from build123d import *

# Parameters (mm, degrees)
F0_W     = 69.85
F0_H     = 101.6
F0_R     = 25.4
F1_DEPTH = 12.7
F2_W     = 69.85
F2_H     = 6.35
F3_DEPTH = 2.54


with BuildPart() as f1:
    # F0 (on Top) → F1 (new body)
    with BuildSketch(Plane.XY):
        Rectangle(F0_W, F0_H)
        Circle(F0_R, mode=Mode.SUBTRACT)
    extrude(amount=F1_DEPTH)

    # F2 (on face) → F3 (cut)
    with BuildSketch(Plane.XY.offset(12.7)):
        with BuildLine():
            Line((-24.8187093164, 5.4029314144), (-34.925, 5.4029314144))
            Line((-34.925, 5.4029314144), (-34.925, 0.3229314144))
            Line((-34.925, 0.3229314144), (-25.3989142655, 0.2348491713))
            ThreePointArc((-25.3989142655, 0.2348491713), (-25.2414282098, 2.8337787368), (-24.8187093164, 5.4029314144))
        make_face()
        with BuildLine():
            Line((-25.3989142655, 0.2348491713), (-34.925, 0.3229314144))
            Line((-34.925, 0.3229314144), (-34.925, -4.7570685856))
            Line((-34.925, -4.7570685856), (-24.9505570774, -4.7570685856))
            ThreePointArc((-24.9505570774, -4.7570685856), (-25.2981644957, -2.2721956671), (-25.3989142655, 0.2348491713))
        make_face()
        with BuildLine():
            Line((34.925, -0.3229314144), (34.925, 5.4029314144))
            Line((34.925, 5.4029314144), (24.8187093164, 5.4029314144))
            ThreePointArc((24.8187093164, 5.4029314144), (25.2542592114, 2.7170557009), (25.4, 0))
            ThreePointArc((25.4, 0), (25.3997285649, -0.1174258405), (25.3989142655, -0.2348491713))
            Line((25.3989142655, -0.2348491713), (34.925, -0.3229314144))
        make_face()
        with BuildLine():
            Line((34.925, -4.7570685856), (34.925, -0.3229314144))
            Line((34.925, -0.3229314144), (25.3989142655, -0.2348491713))
            ThreePointArc((25.3989142655, -0.2348491713), (25.2760743241, -2.5060061383), (24.9505570774, -4.7570685856))
            Line((24.9505570774, -4.7570685856), (34.925, -4.7570685856))
        make_face()
        with Locations((0, 36.0342099249)):
            Rectangle(F2_W, F2_H)
    extrude(amount=-F3_DEPTH, mode=Mode.SUBTRACT)


solid = f1.part
Verification items for the finished model (mm, model axes). A direction names the side the tool comes from. Give positions to 0.01 mm unless a question says otherwise; leave off trailing zeros. Write each loop counter-clockwise with the first axis right and the second up, starting at its lowest first coordinate (ties: lowest second). Pieces come first, ordered by that corner, then holes. Notation, with made-up numbers: M 22.25,29 L 46.25,29 A16 ccw 46.25,38 Z; hole C 19,32 d3. An arc over 180 degrees is marked long. Put each result on its own line as item: value. Start each with the question number.
1. Section check D-D (x = 28.5). Record the cut outline in (y, z), and give its area (3 significant figures).
2. Go/stop test with flat-tipped pins: pin 1 Ø1.5 at (x, y) = (-20.5, -30.5) entering from -Z; pin 2 Ø3 at (x, y) = (27.5, -1) entering from +Z; pin 3 Ø2 at (x, y) = (-2.5, -23.5) entering from -Z. Record where each tip stops, or that it passes through.
3. Scan lines: line 1 along X through (y, z) = (0, 5.75) (3 decimals); line 2 along Y through (x, z) = (-0.5, 5.25); line 3 along Y through (x, z) = (11, 10.25). Record each from-to range of solid material in increasing order. Write a range as [from, to].
4. Draft check along Y on faces 3 (the face through (0, 39.209, 11)), 4 (the face through (0, 28, 12.7)), 5 (the face through (-30, -4.757, 11)), 6 (the face through (0, 50.8, 6)). Enter one of: +Y half, -Y half, draft (parallel to the pull), parting line (faces both ways), or undercut.
5. Set-up check for faces 1 (the face through (0, 32.859, 11)), 2 (the face through (-34.925, -1, 6)): record each of +Z, -Z, +X, -X, +Y, -Y from which the full face is reachable in a straight line by a thin tool's end or side.
6. Section check C-C (z = 8.5). Record the cut outline in (x, y) (3 decimals), and give its area (3 significant figures).
7. Section check B-B (y = -8.5). Record the cut outline in (x, z) (3 decimals).
8. Section check A-A (x = 0). Record the cut outline in (y, z), and give its area (3 significant figures).
Answer list:
1. outline: M -50.8,0 L 50.8,0 L 50.8,12.7 L 39.21,12.7 L 39.21,10.16 L 32.86,10.16 L 32.86,12.7 L 5.4,12.7 L 5.4,10.16 L -4.76,10.16 L -4.76,12.7 L -50.8,12.7 Z
1. area: 1,250 mm2
2. pin 1: z = 0
2. pin 2: z = 10.16
2. pin 3: through
3. line 1: [-34.925, -25.4], [25.4, 34.925]
3. line 2: [-50.8, -25.4], [25.4, 50.8]
3. line 3: [-50.8, -22.89], [22.89, 32.86], [39.21, 50.8]
4. face 3: undercut
4. face 4: draft
4. face 5: undercut
4. face 6: +Y half
5. face 1: +Z, +X, -X
5. face 2: +Z, -Z, -X, +Y, -Y
6. outline: M -34.925,-50.8 L 34.925,-50.8 L 34.925,50.8 L -34.925,50.8 Z; hole C 0,0 d50.8
6. area: 5,070 mm2
7. outline: M -34.925,0 L -23.936,0 L -23.936,12.7 L -34.925,12.7 Z; M 23.936,0 L 34.925,0 L 34.925,12.7 L 23.936,12.7 Z
8. outline: M -50.8,0 L -25.4,0 L -25.4,12.7 L -50.8,12.7 Z; M 25.4,0 L 50.8,0 L 50.8,12.7 L 39.21,12.7 L 39.21,10.16 L 32.86,10.16 L 32.86,12.7 L 25.4,12.7 Z
8. area: 629 mm2
